Build history of the part. All positions in model axes, mm. A direction names the side the tool comes from. Give positions to 0.01 mm unless a question says otherwise; leave off trailing zeros. Loops run counter-clockwise (first coordinate to the right, second up) from the corner with the lowest first, then second, coordinate; pieces in that order, holes last. Notation, with made-up numbers: (4, -23.5) -> (63, -23.5) arc R33 cw to (63, 10.5) -> close; hole circle Ø11 at (64.5, 68.5). An arc over 180 degrees is marked (long way). One line per question, with ' | ' between items. Start each with the question number.
(1) 3-axis set-ups, long thin cutter, end or side, ignore diameter. For faces 1 (the face through (50, 10, 2)), 2 (the face through (117.948, -6.111, 1.972)): which of +Z, -Z, +X, -X, +Y, -Y reach the whole face in a straight line?
(2) Mould opens along Y. For faces 3 (the face through (49, -19, 2)), 4 (the face through (108.401, 16.996, 1.972)), 5 (the face through (95.904, -0.18, 1.972)) say: pulls with the +Y half, pulls with the -Y half, needs draft (parallel to the pull), parting line crosses it, or undercut.
(3) Slice it at B-B, the plane x = 31.5. Write the cut outline in (y, z), then the cut area to 3 significant figures.
(4) Drill centre lines: L1, parallel to Y at x = 84, z = 1.8; L2, parallel to Y at x = 67, z = 0.4; L3, parallel to Y at x = 15, z = 0.9. Where is each one in solid material? Low to high. Write a range as from..to.
(5) Flat gauge pin, fed straight in: pin 1 Ø2 at (y, z) = (5, 2) entering from -X. Where does the tip first touch, or does it go through?
(6) Slice it at C-C, the plane z = 1.95. Give the number of separate pieces and of enclosed holes in the cut face, then the cut area to 3 significant figures.
(7) Slice it at A-A, the plane x = 84. Write the cut outline in (y, z), then the cut area to 3 significant figures.
Solid Edge part; units mm, degrees
sketch "Sketch1" plane through (0, 0, 0) normal (0, 0, 1) x (1, 0, 0)
  line L0 (100, -19) -> (102.48, -18.8375)
  line L1 (102.48, -18.8375) -> (104.9176, -18.3526)
  line L2 (104.9176, -18.3526) -> (107.271, -17.5537)
  line L3 (107.271, -17.5537) -> (109.5, -16.4545)
  line L4 (109.5, -16.4545) -> (111.5665, -15.0737)
  line L5 (111.5665, -15.0737) -> (113.435, -13.435)
  line L6 (113.435, -13.435) -> (115.0737, -11.5665)
  line L7 (115.0737, -11.5665) -> (116.4545, -9.5)
  line L8 (116.4545, -9.5) -> (117.5537, -7.271)
  line L9 (117.5537, -7.271) -> (118.3526, -4.9176)
  line L10 (118.3526, -4.9176) -> (118.8375, -2.48)
  line L11 (118.8375, -2.48) -> (119, 0)
  line L12 (119, 0) -> (118.8375, 2.48)
  line L13 (118.8375, 2.48) -> (118.3526, 4.9176)
  line L14 (118.3526, 4.9176) -> (117.5537, 7.271)
  line L15 (117.5537, 7.271) -> (116.4545, 9.5)
  line L16 (116.4545, 9.5) -> (115.0737, 11.5665)
  line L17 (115.0737, 11.5665) -> (113.435, 13.435)
  line L18 (113.435, 13.435) -> (111.5665, 15.0737)
  line L19 (111.5665, 15.0737) -> (109.5, 16.4545)
  line L20 (109.5, 16.4545) -> (107.271, 17.5537)
  line L21 (107.271, 17.5537) -> (104.9176, 18.3526)
  line L22 (104.9176, 18.3526) -> (102.48, 18.8375)
  line L23 (102.48, 18.8375) -> (100, 19)
  line L24 (100, 19) -> (0, 19)
  line L25 (0, 19) -> (-2.48, 18.8375)
  line L26 (-2.48, 18.8375) -> (-4.9176, 18.3526)
  line L27 (-4.9176, 18.3526) -> (-7.271, 17.5537)
  line L28 (-7.271, 17.5537) -> (-9.5, 16.4545)
  line L29 (-9.5, 16.4545) -> (-11.5665, 15.0737)
  line L30 (-11.5665, 15.0737) -> (-13.435, 13.435)
  line L31 (-13.435, 13.435) -> (-15.0737, 11.5665)
  line L32 (-15.0737, 11.5665) -> (-16.4545, 9.5)
  line L33 (-16.4545, 9.5) -> (-17.5537, 7.271)
  line L34 (-17.5537, 7.271) -> (-18.3526, 4.9176)
  line L35 (-18.3526, 4.9176) -> (-18.8375, 2.48)
  line L36 (-18.8375, 2.48) -> (-19, 0)
  line L37 (-19, 0) -> (-18.8375, -2.48)
  line L38 (-18.8375, -2.48) -> (-18.3526, -4.9176)
  line L39 (-18.3526, -4.9176) -> (-17.5537, -7.271)
  line L40 (-17.5537, -7.271) -> (-16.4545, -9.5)
  line L41 (-16.4545, -9.5) -> (-15.0737, -11.5665)
  line L42 (-15.0737, -11.5665) -> (-13.435, -13.435)
  line L43 (-13.435, -13.435) -> (-11.5665, -15.0737)
  line L44 (-11.5665, -15.0737) -> (-9.5, -16.4545)
  line L45 (-9.5, -16.4545) -> (-7.271, -17.5537)
  line L46 (-7.271, -17.5537) -> (-4.9176, -18.3526)
  line L47 (-4.9176, -18.3526) -> (-2.48, -18.8375)
  line L48 (-2.48, -18.8375) -> (0, -19)
  line L49 (0, -19) -> (100, -19)
  circle A0 centre (0, 0) radius 4.1
  circle A1 centre (100, 0) radius 4.1
  line L50 (27, -10) -> (73, -10)
  line L51 (73, -10) -> (73, 10)
  line L52 (73, 10) -> (27, 10)
  line L53 (27, 10) -> (27, -10)
  circle A2 centre (16, -12) radius 1.7
  circle A3 centre (16, 12) radius 1.7
  circle A4 centre (84, -12) radius 1.7
  circle A5 centre (84, 12) radius 1.7
extrude "Protrusion1" add sketch "Sketch1" along normal blind 4
Final values:
1) face 1: +Z, -Z | face 2: +Z, -Z, +X, -Y
2) face 3: pulls with the -Y half | face 4: pulls with the +Y half | face 5: undercut
3) outline: (-19, 0) -> (-10, 0) -> (-10, 4) -> (-19, 4) -> close; (10, 0) -> (19, 0) -> (19, 4) -> (10, 4) -> close | area: 72.0 mm2
4) L1: -19..-13.7, -10.3..10.3, 13.7..19 | L2: -19..-10, 10..19 | L3: -19..-13.37, -10.63..10.63, 13.37..19
5) pin 1: x = -18.54
6) separate pieces: 1 | enclosed holes: 7 | area: 3,870 mm2
7) outline: (-19, 0) -> (-13.7, 0) -> (-13.7, 4) -> (-19, 4) -> close; (-10.3, 0) -> (10.3, 0) -> (10.3, 4) -> (-10.3, 4) -> close; (13.7, 0) -> (19, 0) -> (19, 4) -> (13.7, 4) -> close | area: 125 mm2
